Geometry: final body of the model. Coordinates: model frame, mm. A direction names the side the tool comes from. Round coordinates to 2 decimals unless told otherwise and drop trailing zeros. Loops run counter-clockwise (first coordinate to the right, second up) from the corner with the lowest first, then second, coordinate; pieces in that order, holes last. Notation, with made-up numbers: (32.5, 38.25) -> (53.5, 38.25) arc R16 ccw to (53.5, 67.25) -> close; hole circle Ø4 at (-20, -5.75). An arc over 180 degrees is marked (long way). Answer in a Markdown table with one row per item.
```python
from build123d import *

# Parameters (mm, degrees)
SKETCH1_W           = 45
SKETCH1_H           = 10
BOSS_EXTRUDE1_DEPTH = 10
SKETCH2_W           = 10
SKETCH2_H           = 5
BOSS_EXTRUDE2_DEPTH = 10
SKETCH3_W           = 10
SKETCH3_H           = 5
BOSS_EXTRUDE3_DEPTH = 10
SKETCH4_R           = 1.5
CUT_EXTRUDE1_DEPTH  = 5
SKETCH5_R           = 1.5
CUT_EXTRUDE2_DEPTH  = 5
SKETCH6_R           = 1.5
CUT_EXTRUDE3_DEPTH  = 5
CUT_EXTRUDE4_START  = -5
SKETCH7_R           = 1.5
CUT_EXTRUDE4_DEPTH  = 5
SKETCH8_R           = 1.5
CUT_EXTRUDE5_DEPTH  = 5
SKETCH9_R           = 1.5
CUT_EXTRUDE6_DEPTH  = 5


with BuildPart() as part:
    # Sketch1 → Boss-Extrude1 (new body)
    with BuildSketch(Plane.XY):
        with Locations((22.5, 5)):
            Rectangle(SKETCH1_W, SKETCH1_H)
    extrude(amount=BOSS_EXTRUDE1_DEPTH)

    # Sketch2 → Boss-Extrude2 (add)
    with BuildSketch(Plane(origin=(0, 10, 0), x_dir=(1, 0, 0), z_dir=(0, 1, 0))):
        with Locations((5, -2.5)):
            Rectangle(SKETCH2_W, SKETCH2_H)
        with Locations((40, -2.5)):
            Rectangle(SKETCH2_W, SKETCH2_H)
    extrude(amount=BOSS_EXTRUDE2_DEPTH)

    # Sketch3 → Boss-Extrude3 (add)
    with BuildSketch(Plane.XY.offset(10)):
        with Locations((5, 2.5)):
            Rectangle(SKETCH3_W, SKETCH3_H)
        with Locations((40, 2.5)):
            Rectangle(SKETCH3_W, SKETCH3_H)
    extrude(amount=BOSS_EXTRUDE3_DEPTH)

    # Sketch4 → Cut-Extrude1 (cut)
    with BuildSketch(Plane.ZY):
        with Locations((5, 5)):
            Circle(SKETCH4_R)
    extrude(amount=-CUT_EXTRUDE1_DEPTH, mode=Mode.SUBTRACT)

    # Sketch5 → Cut-Extrude2 (cut)
    with BuildSketch(Plane.XY.offset(5)):
        with Locations((5, 15)):
            Circle(SKETCH5_R)
    extrude(amount=-CUT_EXTRUDE2_DEPTH, mode=Mode.SUBTRACT)

    # Sketch6 → Cut-Extrude3 (cut)
    with BuildSketch(Plane(origin=(0, 5, 0), x_dir=(1, 0, 0), z_dir=(0, 1, 0))):
        with Locations(Location((5, -15, 0), (0, 0, 270))):
            Circle(SKETCH6_R)
    extrude(amount=-CUT_EXTRUDE3_DEPTH, mode=Mode.SUBTRACT)

    # Sketch7 → Cut-Extrude4 (cut)
    with BuildSketch(Plane(origin=(45, 0, 0), x_dir=(0, 0, -1), z_dir=(1, 0, 0)).offset(CUT_EXTRUDE4_START)):
        with Locations(Location((-5, 5, 0), (0, 0, 180))):
            Circle(SKETCH7_R)
    extrude(amount=CUT_EXTRUDE4_DEPTH, mode=Mode.SUBTRACT)

    # Sketch8 → Cut-Extrude5 (cut)
    with BuildSketch(Plane.XY.offset(5)):
        with Locations((40, 15)):
            Circle(SKETCH8_R)
    extrude(amount=-CUT_EXTRUDE5_DEPTH, mode=Mode.SUBTRACT)

    # Sketch9 → Cut-Extrude6 (cut)
    with BuildSketch(Plane(origin=(0, 5, 0), x_dir=(1, 0, 0), z_dir=(0, 1, 0))):
        with Locations(Location((40, -15, 0), (0, 0, 180))):
            Circle(SKETCH9_R)
    extrude(amount=-CUT_EXTRUDE6_DEPTH, mode=Mode.SUBTRACT)


solid = part.part
```
Item 1: Pin query (flat end, axial travel): pin 1 Ø2.5 at (y, z) = (5, 5) entering from -X; pin 2 Ø1 at (x, z) = (35.5, 14.5) entering from +Y; pin 3 Ø1.5 at (y, z) = (5.5, 5.5) entering from +X. Return the tip coordinate at first contact, or that it passes through.
Answer:
| item | result |
|---|---|
| pin 1 | stops at x = 5 |
| pin 2 | stops at y = 5 |
| pin 3 | stops at x = 40 |
Item 2: Cut plane C-C (y = 14.25). Output: boundary loops of the cut face in (x, z).
Answer:
| item | result |
|---|---|
| outline | (0, 0) -> (3.7, 0) -> (3.7, 5) -> (0, 5) -> close; (6.3, 0) -> (10, 0) -> (10, 5) -> (6.3, 5) -> close; (35, 0) -> (38.7, 0) -> (38.7, 5) -> (35, 5) -> close; (41.3, 0) -> (45, 0) -> (45, 5) -> (41.3, 5) -> close |
Item 3: Draft query along X for faces 5 (the face through (40, 5, 5)), 6 (the face through (22, 0, 8)), 7 (the face through (10, 2, 15)). Return one class per face: pulls with the +X half, pulls with the -X half, needs draft (parallel to the pull), parting line crosses it, or undercut.
Answer:
| item | result |
|---|---|
| face 5 | pulls with the +X half |
| face 6 | needs draft |
| face 7 | undercut |
Item 4: Line query: probe 1 along X at (y, z) = (11, 1); probe 2 along X at (y, z) = (1.5, 14); probe 3 along Z at (x, y) = (40, 3). Output: solid intervals per line, ascending. Write a range as [from, to].
Answer:
| item | result |
|---|---|
| probe 1 | x = [0, 10], [35, 45] |
| probe 2 | x = [0, 3.88], [6.12, 10], [35, 38.88], [41.12, 45] |
| probe 3 | z = [0, 13.5], [16.5, 20] |
Item 5: Reachability of faces 1 (the face through (35, 15, 3)), 2 (the face through (35, 2, 15)), 3 (the face through (42.46, 4.55, 6.43)), 4 (the face through (3.8, 5, 13.8)) from +Z, -Z, +X, -X, +Y, -Y: full face, straight path, thin tool, end or side. Return the list, or none.
Answer:
| item | result |
|---|---|
| face 1 | +Z, -Z, +Y |
| face 2 | +Z, +Y, -Y |
| face 3 | +X |
| face 4 | +Z, +X, -X, +Y |
Item 6: Cut plane B-B (x = 4.5). Output: boundary loops of the cut face in (y, z), then the cut area to 3 significant figures.
Answer:
| item | result |
|---|---|
| outline | (0, 0) -> (13.59, 0) -> (13.59, 5) -> (10, 5) -> (10, 10) -> (5, 10) -> (5, 13.59) -> (0, 13.59) -> close; (0, 16.41) -> (5, 16.41) -> (5, 20) -> (0, 20) -> close; (16.41, 0) -> (20, 0) -> (20, 5) -> (16.41, 5) -> close; hole circle Ø3 at (5, 5) |
| area | 165 mm² |
Item 7: Cut plane A-A (z = 11.75). Output: boundary loops of the cut face in (x, y), then the cut area to 3 significant figures.
Answer:
| item | result |
|---|---|
| outline | (0, 0) -> (10, 0) -> (10, 5) -> (0, 5) -> close; (35, 0) -> (45, 0) -> (45, 5) -> (35, 5) -> close |
| area | 100 mm² |
Item 8: Cut plane D-D (z = 15). Output: boundary loops of the cut face in (x, y).
Answer:
| item | result |
|---|---|
| outline | (0, 0) -> (3.5, 0) -> (3.5, 5) -> (0, 5) -> close; (6.5, 0) -> (10, 0) -> (10, 5) -> (6.5, 5) -> close; (35, 0) -> (38.5, 0) -> (38.5, 5) -> (35, 5) -> close; (41.5, 0) -> (45, 0) -> (45, 5) -> (41.5, 5) -> close |
